```python
from build123d import *

# Parameters (mm, degrees)
ESTRUSIONE_ESTRUSIONE1_DEPTH = 10
ESTRUSIONE_ESTRUSIONE2_DEPTH = 40
ESTRUSIONE_ESTRUSIONE3_START = 20
SCHIZZO2_3_R                 = 10
ESTRUSIONE_ESTRUSIONE3_DEPTH = 20
FORO_10_0_10_1_D             = 10
FORO_10_0_10_1_DEPTH         = 45
FORO_8_0_8_1_D               = 8
RACCORDO1_R                  = 5
RACCORDO2_R                  = 5


with BuildPart() as part:
    # Schizzo1 → Estrusione-Estrusione1 (new body)
    with BuildSketch(Plane.XY):
        with BuildLine():
            Line((41.339745962, -13.867513459), (8.660254038, 42.735026919))
            ThreePointArc((8.660254038, 42.735026919), (0, 47.735026919), (-8.660254038, 42.735026919))
            Line((-8.660254038, 42.735026919), (-41.339745962, -13.867513459))
            ThreePointArc((-41.339745962, -13.867513459), (-41.339745962, -23.867513459), (-32.679491924, -28.867513459))
            Line((-32.679491924, -28.867513459), (32.679491924, -28.867513459))
            ThreePointArc((32.679491924, -28.867513459), (41.339745962, -23.867513459), (41.339745962, -13.867513459))
        make_face()
    extrude(amount=ESTRUSIONE_ESTRUSIONE1_DEPTH)

    # Schizzo2 → Estrusione-Estrusione2 (add)
    with BuildSketch(Plane.XZ.offset(28.867513459)):
        with BuildLine():
            Line((-10, 10), (10, 10))
            Line((10, 10), (10, 20))
            ThreePointArc((10, 20), (0, 30), (-10, 20))
            Line((-10, 20), (-10, 10))
        make_face()
    extrude(amount=-ESTRUSIONE_ESTRUSIONE2_DEPTH)

    # Schizzo2_3 → Estrusione-Estrusione3 (add)
    with BuildSketch(Plane.XZ.offset(28.867513459).offset(ESTRUSIONE_ESTRUSIONE3_START)):
        with Locations((0, 20)):
            Circle(SCHIZZO2_3_R)
    extrude(amount=-ESTRUSIONE_ESTRUSIONE3_DEPTH)

    # Foro _10.0 _10_-1
    with Locations(Plane(origin=(0, -48.867513459, 0), x_dir=(-1, 0, 0), z_dir=(0, -1, 0))):
        with Locations((0, -20)):
            Hole(FORO_10_0_10_1_D / 2, depth=FORO_10_0_10_1_DEPTH)

    # Foro _8.0 _8_-1 (through all)
    with Locations(Plane.XY.offset(10)):
        with Locations((0, 37.735026919), (-32.679491924, -18.867513459), (32.679491924, -18.867513459)):
            Hole(FORO_8_0_8_1_D / 2)

    # Raccordo1
    raccordo1_edges = [part.edges().sort_by_distance(p)[0] for p in [
        (0, 11.132486541, 30),
        (10, 11.132486541, 15),
        (-10, 11.132486541, 15),
    ]]
    fillet(raccordo1_edges, radius=RACCORDO1_R)

    # Raccordo2
    raccordo2_edges = [part.edges().sort_by_distance(p)[0] for p in [
        (10, -11.367513459, 10),
        (0, 11.132486541, 10),
        (-10, -11.367513459, 10),
        (8.535533906, 9.668020446, 10),
        (-8.535533906, 9.668020446, 10),
    ]]
    fillet(raccordo2_edges, radius=RACCORDO2_R)


solid = part.part
```
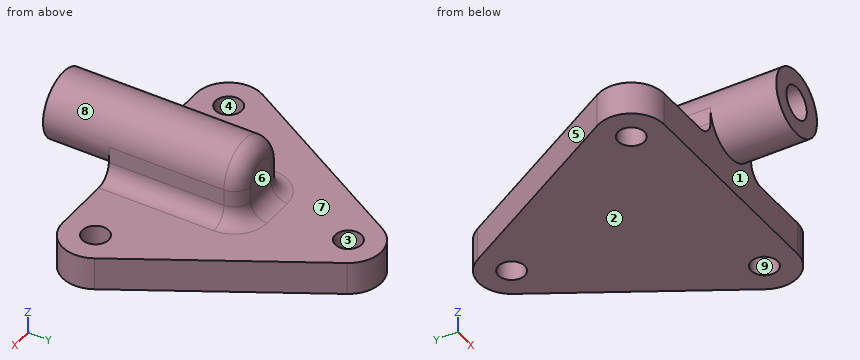
Here's how the part is built. I have some questions about the finished solid (model axes, mm). Face numbers are marked on the shaded views. A direction names the side the tool comes from. Give positions to 0.01 mm unless a question says otherwise; leave off trailing zeros. Loops run counter-clockwise (first coordinate to the right, second up) from the corner with the lowest first, then second, coordinate; pieces in that order, holes last. Notation, with made-up numbers: M 84,4.5 L 125,4.5 A17 cw 125,15.5 Z; hole C 1.25,81.25 d8. An arc over 180 degrees is marked long. Put each result on its own line as item: value. Start each with the question number.
(1) I want a section at C-C on y = -24. Please give me the cut outline in (x, z), then the cut area to 3 significant figures.
(2) For the marked faces 5, 6, 7, 8 and 9, which set-ups out of +Z, -Z, +X, -X, +Y, -Y let a thin tool reach every point of the face, with its end or its side?
(3) I need wall thicknesses on line 1 along X through (y, z) = (-17, 20); line 2 along Z through (x, y) = (0, -35); line 3 along Z through (x, y) = (0, -23). Which ranges of each line are inside material? Lowest first, please. Write a range as [from, to].
(4) Will these pins go through, and if not, where does the flat tip stop? pin 1 Ø13 at (x, y) = (0, 37.74) entering from +Z; pin 2 Ø5.5 at (y, z) = (-5, 16.5) entering from -X; pin 3 Ø2.5 at (y, z) = (-10.5, 18.5) entering from +X; pin 4 Ø8 at (x, y) = (18, -36.5) entering from +Z.
(5) I want a section at A-A on y = -39. Please give me the cut outline in (x, z).
(6) If we mould it in two halves opening along Y, with no side actions, what happens to the marked faces 1, 2, 3 and 4? For each: +Y half, -Y half, draft (parallel to the pull), parting line (faces both ways), or undercut.
(7) I want a section at D-D on x = 17. Please give me the cut outline in (y, z).
(8) I want a section at B-B on z = 12.25. Please give me the cut outline in (x, y), then the cut area to 3 significant figures.
Answer block:
1. outline: M -41.26,0 L 41.26,0 L 41.26,10 L 15,10 A5 cw 10,15 L 10,20 A10 ccw -10,20 L -10,15 A5 cw -15,10 L -41.26,10 Z; hole C 0,20 d10
1. area: 1,110 mm^2
2. face 5: +Z, -Z, -X, +Y
2. face 6: +Z, +X, -X, +Y
2. face 7: +Z, +Y
2. face 8: -Y
2. face 9: +Z, -Z
3. line 1: [-10, -5], [5, 10]
3. line 2: [10, 15], [25, 30]
3. line 3: [0, 15], [25, 30]
4. pin 1: z = 10
4. pin 2: x = -10.16
4. pin 3: x = 10
4. pin 4: through
5. outline: C 0,20 d20; hole C 0,20 d10
6. face 1: -Y half
6. face 2: draft
6. face 3: undercut
6. face 4: undercut
7. outline: M -28.87,0 L 28.29,0 L 28.29,10 L -28.87,10 Z
8. outline: M -10.82,-28.87 L -6.32,-28.87 L -6.32,-48.87 L 6.32,-48.87 L 6.32,-28.87 L 10.82,-28.87 L 10.82,6.13 A5.82 ccw 5,11.96 L -5,11.96 A5.82 ccw -10.82,6.13 Z
8. area: 1,120 mm^2
